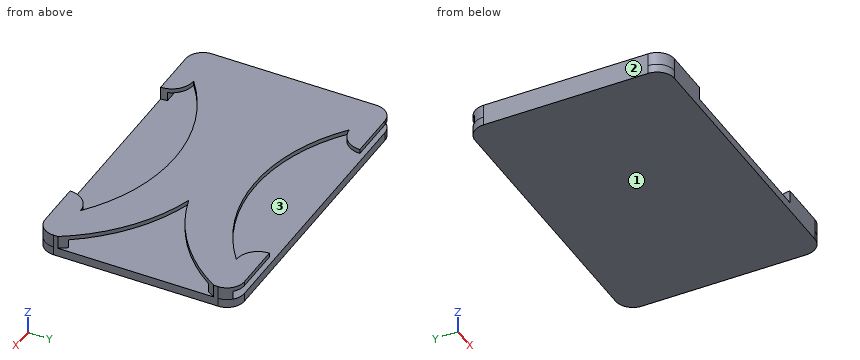
```python
from build123d import *

# Parameters (mm, degrees)
F0_W     = 88.9
F0_H     = 58.42
F1_DEPTH = 2.54
F2_R     = 5.08
F4_DEPTH = 3.81
F5_W     = 86.106
F5_H     = 63.5
F6_DEPTH = 2.54


with BuildPart() as f1:
    # F0 (on Top) → F1 (new body)
    with BuildSketch(Plane.XY):
        with Locations((-15.937483, -2.926046)):
            Rectangle(F0_W, F0_H)
    extrude(amount=F1_DEPTH)

    # F2
    f2_edges = [f1.edges().sort_by_distance(p)[0] for p in [
        (-60.387483, 26.283954, 1.27),
        (-60.387483, -32.136046, 1.27),
        (28.512517, -32.136046, 1.27),
        (28.512517, 26.283954, 1.27),
    ]]
    fillet(f2_edges, radius=F2_R)

    # F3 (on face) → F4 (join)
    with BuildSketch(Plane.XY.offset(2.54)):
        with BuildLine():
            ThreePointArc((-55.307483, 26.283954), (-58.899585, 24.796056), (-60.387483, 21.203954))
            Line((-60.387483, 21.203954), (-60.387483, 19.933954))
            ThreePointArc((-60.387483, 19.933954), (-47.671274, 5.737441), (-30.695205, -2.926046))
            ThreePointArc((-30.695205, -2.926046), (-47.671274, -11.589534), (-60.387483, -25.786046))
            Line((-60.387483, -25.786046), (-60.387483, -27.056046))
            ThreePointArc((-60.387483, -27.056046), (-58.899585, -30.648149), (-55.307483, -32.136046))
            Line((-55.307483, -32.136046), (-41.337483, -32.136046))
            ThreePointArc((-41.337483, -32.136046), (-43.197355, -27.645918), (-47.687483, -25.786046))
            ThreePointArc((-47.687483, -25.786046), (-15.937483, -14.641784), (15.812517, -25.786046))
            ThreePointArc((15.812517, -25.786046), (11.322389, -27.645918), (9.462517, -32.136046))
            Line((9.462517, -32.136046), (23.432517, -32.136046))
            ThreePointArc((23.432517, -32.136046), (27.02462, -30.648149), (28.512517, -27.056046))
            Line((28.512517, -27.056046), (28.512517, -25.786046))
            ThreePointArc((28.512517, -25.786046), (15.796308, -11.589534), (-1.17976, -2.926046))
            ThreePointArc((-1.17976, -2.926046), (15.796308, 5.737441), (28.512517, 19.933954))
            Line((28.512517, 19.933954), (28.512517, 21.203954))
            ThreePointArc((28.512517, 21.203954), (27.02462, 24.796056), (23.432517, 26.283954))
            Line((23.432517, 26.283954), (9.462517, 26.283954))
            ThreePointArc((9.462517, 26.283954), (11.322389, 21.793825), (15.812517, 19.933954))
            ThreePointArc((15.812517, 19.933954), (-15.937483, 8.789691), (-47.687483, 19.933954))
            ThreePointArc((-47.687483, 19.933954), (-43.197355, 21.793825), (-41.337483, 26.283954))
            Line((-41.337483, 26.283954), (-55.307483, 26.283954))
        make_face()
        with BuildLine():
            ThreePointArc((-30.695205, -2.926046), (-47.671274, 5.737441), (-60.387483, 19.933954))
            Line((-60.387483, 19.933954), (-60.387483, -25.786046))
            ThreePointArc((-60.387483, -25.786046), (-47.671274, -11.589534), (-30.695205, -2.926046))
        make_face()
    extrude(amount=F4_DEPTH)

    # F5 (on face) → F6 (cut)
    with BuildSketch(Plane.XY.offset(2.54)):
        with Locations((-16.064483, 1.518954)):
            Rectangle(F5_W, F5_H)
    extrude(amount=F6_DEPTH, mode=Mode.SUBTRACT)


solid = f1.part
```
The listing builds one solid part. Answer for the finished solid, in the listing's coordinates (mm). Face numbers are marked on the shaded views. Coordinates: 2 decimals unless noted, no trailing zeros. Write each loop counter-clockwise with the first axis right and the second up, starting at its lowest first coordinate (ties: lowest second). Pieces come first, ordered by that corner, then holes. Notation, with made-up numbers: (-2, 77) - (40, 77) arc R33 ccw to (40, 112) - close; hole circle Ø5 at (-8.75, -26.5). An arc over 180 degrees is marked (long way). One line per item, written item: value.
1) Find section A-A (y = 10). Give the vertices of the cut face in (x, z), and give its area (3 significant figures).
Geometry check:
outline: (-60.39, 0) - (28.51, 0) - (28.51, 2.54) - (-59.12, 2.54) - (-59.12, 5.08) - (-26.96, 5.08) - (-26.96, 6.35) - (-60.39, 6.35) - close; (-4.91, 5.08) - (20.67, 5.08) - (20.67, 6.35) - (-4.91, 6.35) - close
area: 304 mm2
2) Find section B-B (x = -12). Give the vertices of the cut face in (y, z).
Geometry check:
outline: (-32.14, 0) - (26.28, 0) - (26.28, 2.54) - (-32.14, 2.54) - close; (-14.79, 5.08) - (8.94, 5.08) - (8.94, 6.35) - (-14.79, 6.35) - close
3) For a pull along Z with two mould halves and no side action, classify the marked faces 1, 2 and 3 as pulls with the +Z half, pulls with the -Z half, needs draft (parallel to the pull), parting line crosses it, or undercut.
Geometry check:
face 1: pulls with the -Z half
face 2: needs draft
face 3: undercut
4) Consider line 1 along Z through (x, y) = (-4.5, -2); line 2 along Y through (x, z) = (-52, 3.25); line 3 along Y through (x, z) = (-46.5, 6.25). Determine where each line is inside the solid, lowest interval first. Write a range as from..to.
Geometry check:
line 1: z = 0..2.54, 5.08..6.35
line 2: y = -32.14..-30.23
line 3: y = -32.14..-25.9, -24.86..19.01, 20.05..26.28
5) Find section C-C (x = 13). Give the vertices of the cut face in (y, z), and give its area (3 significant figures).
Geometry check:
outline: (-32.14, 0) - (26.28, 0) - (26.28, 2.54) - (-30.23, 2.54) - (-30.23, 5.08) - (-26.44, 5.08) - (-26.44, 6.35) - (-32.14, 6.35) - close; (-23.69, 5.08) - (-9.58, 5.08) - (-9.58, 6.35) - (-23.69, 6.35) - close; (3.73, 5.08) - (17.84, 5.08) - (17.84, 6.35) - (3.73, 6.35) - close; (20.59, 5.08) - (26.28, 5.08) - (26.28, 6.35) - (20.59, 6.35) - close
area: 204 mm2
6) Find section D-D (y = -10.5). Give the vertices of the cut face in (x, z), and give its area (3 significant figures).
Geometry check:
outline: (-60.39, 0) - (28.51, 0) - (28.51, 2.54) - (-59.12, 2.54) - (-59.12, 5.08) - (14.33, 5.08) - (14.33, 6.35) - (-60.39, 6.35) - close
area: 324 mm2
7) Each of these flat-tipped pins is pushed along its axis until it touches: pin 1 Ø1.3 at (y, z) = (-28.5, 3) entering from -X; pin 2 Ø0.8 at (x, z) = (21.5, 3.5) entering from +Y. Where does it stop, or does it pass through?
Geometry check:
pin 1: stops at x = -60.33
pin 2: stops at y = -30.23
